```python
from build123d import *

# Parameters (mm, degrees)
SKETCH1_W           = 15
SKETCH1_H           = 13
BOSS_EXTRUDE1_DEPTH = 3
BOSS_EXTRUDE1_TAPER = 25
SKETCH2_W           = 7
SKETCH2_H           = 6
BOSS_EXTRUDE2_DEPTH = 3
SKETCH4_W           = 13
SKETCH4_H           = 11
BOSS_EXTRUDE3_DEPTH = 2


with BuildPart() as part:
    # Sketch1 → Boss-Extrude1 (new body)
    with BuildSketch(Plane(origin=(0, 0, 0), x_dir=(1, 0, 0), z_dir=(0, 1, 0))):
        with Locations((-1.976635514, -0.911214953)):
            Rectangle(SKETCH1_W, SKETCH1_H)
    extrude(amount=BOSS_EXTRUDE1_DEPTH, taper=BOSS_EXTRUDE1_TAPER)

    # Sketch2 → Boss-Extrude2 (add)
    with BuildSketch(Plane(origin=(0, 3, 0), x_dir=(1, 0, 0), z_dir=(0, 1, 0))):
        with Locations((-1.761302023, -0.89583399)):
            Rectangle(SKETCH2_W, SKETCH2_H)
    extrude(amount=BOSS_EXTRUDE2_DEPTH)

    # Sketch4 → Boss-Extrude3 (add)
    with BuildSketch(Plane.XZ):
        with Locations((-1.976635514, 0.911214953)):
            Rectangle(SKETCH4_W, SKETCH4_H)
    extrude(amount=BOSS_EXTRUDE3_DEPTH)


solid = part.part
```
Input: part model. Units: mm. Frame: model coordinates. A direction names the side the tool comes from. Give positions to 0.01 mm unless a question says otherwise; leave off trailing zeros. Order: outer loops, then holes, each group sorted by start corner. A loop starts at its lowest first (then second) coordinate and runs counter-clockwise, first axis right, second up. Notation, with made-up numbers: (4, -17) - (17, -17) arc R15 cw to (17, -5) - close; hole circle Ø10 at (73.5, 11). An arc over 180 degrees is marked (long way). Use a Markdown table: item, result.
(1) Section query B-B (y = 5.5). Output: boundary loops of the cut face in (x, z).
Computed values:
| item | result |
|---|---|
| outline | (-5.26, -2.1) - (1.74, -2.1) - (1.74, 3.9) - (-5.26, 3.9) - close |
(2) Access query for faces 1 (the flat face through (-2, 4, 3.896)), 2 (the flat face through (-2, 4, -2.104)), 3 (the flat face through (1.739, 4, 1)). Directions: +Z, -Z, +X, -X, +Y, -Y. A direction counts if a zero-diameter tool reaches every point of the face in a straight line with its end or side. Return the directions, or none.
Computed values:
| item | result |
|---|---|
| face 1 | +Z, +X, -X, +Y |
| face 2 | -Z, +X, -X, +Y |
| face 3 | +Z, -Z, +X, +Y |
(3) Section query A-A (y = -1). Output: boundary loops of the cut face in (x, z).
Computed values:
| item | result |
|---|---|
| outline | (-8.48, -4.59) - (4.52, -4.59) - (4.52, 6.41) - (-8.48, 6.41) - close |
(4) Line query: line 1 (Z direction, x = 0.5, y = 4.5); line 2 (Z direction, x = -3.5, y = -0.5); line 3 (Y direction, x = -5.5, z = -3.25). Output: solid intervals per line, ascending. Write a range as from..to.
Computed values:
| item | result |
|---|---|
| line 1 | z = -2.1..3.9 |
| line 2 | z = -4.59..6.41 |
| line 3 | y = -2..3 |
(5) Pin query (flat end, axial travel): pin 1 (1.5 mm diameter, centred on y = 4.5, z = 2, fed in from -X); pin 2 (1.6 mm diameter, centred on x = -2.5, y = -0.5, fed in from +Z); pin 3 (0.6 mm diameter, centred on y = -1.5, z = 1.5, fed in from +X). Return the tip coordinate at first contact, or that it passes through.
Computed values:
| item | result |
|---|---|
| pin 1 | stops at x = -5.26 |
| pin 2 | stops at z = 7.41 |
| pin 3 | stops at x = 4.52 |
